Design review of the part built by this model. Coordinates are the model's own, in mm. A direction names the side the tool comes from. Coordinates: 2 decimals unless noted, no trailing zeros. Loops run counter-clockwise (first coordinate to the right, second up) from the corner with the lowest first, then second, coordinate; pieces in that order, holes last. Notation, with made-up numbers: (13, 22.25) - (55, 22.25) arc R34 cw to (55, 55.25) - close; hole circle Ø8 at (43.5, -13.75). An arc over 180 degrees is marked (long way). Answer in a Markdown table with one row per item. Add a question column.
(1) To check wall thickness, follow L1, parallel to Y at x = 82, z = 45.5; L2, parallel to Y at x = -76, z = 28; L3, parallel to Z at x = 85, y = -9.5. State the ranges of each line that lie inside material, in increasing order. Write a range as [from, to].
(2) The part is to be moulded in two halves that separate along X. For faces 3 (the face through (-53.978, -5.67, -133.786)), 4 (the face through (-79.557, 3.451, -113.968)), 5 (the face through (-113, 0, 112)), 6 (the face through (55.637, -5.67, 110.036)), say which applies: released by +X, released by -X, zero draft, split by the parting line, or undercut.
(3) We need section A-A, the plane y = 3.5. Write out the cut boundary in (x, z), plus the area to 3 significant figures.
(4) For faces 1 (the face through (-78, 0, -2)), 2 (the face through (-55, 8, 34)), list the 3-axis set-ups (+Z, -Z, +X, -X, +Y, -Y) from which the entire face can be reached by the end or side of a thin tool; tool diameter is ignored.
(5) Clearance check with flat-ended pins moving along their axes: pin 1 (1 mm diameter, centred on y = -8, z = 42, fed in from -X); pin 2 (8 mm diameter, centred on y = 4.5, z = 80, fed in from -X); pin 3 (4 mm diameter, centred on y = -7.5, z = 12.5, fed in from -X); pin 4 (11.5 mm diameter, centred on x = -53.13, z = -140.23, fed in from +Y). State where each tip first meets the part, or that it passes through.
from build123d import *

# Parameters (mm, degrees)
F0_R     = 160
F0_R_2   = 6.5
F0_R_3   = 36
F1_DEPTH = 11.5
F2_SIZE  = 1
F3_R     = 122
F3_R_2   = 36
F3_R_3   = 25.5
F4_DEPTH = 8
F5_SIZE  = 1


with BuildPart() as f1:
    # F0 (on Front) → F1 (new body)
    with BuildSketch(Plane.XZ):
        with Locations((-53.132202721, 5.1132893958)):
            Circle(F0_R)
        with Locations((-155.6978265414, -97.8607830485)):
            Circle(F0_R_2, mode=Mode.SUBTRACT)
        with Locations((-53.132202721, -140.2307106042)):
            Circle(F0_R_2, mode=Mode.SUBTRACT)
        with Locations((49.4334210995, -97.8607830485)):
            Circle(F0_R_2, mode=Mode.SUBTRACT)
        with Locations((90.8079806329, 5.1103962891)):
            Circle(F0_R_2, mode=Mode.SUBTRACT)
        with Locations((-197.0651851107, 5.1132893958)):
            Circle(F0_R_2, mode=Mode.SUBTRACT)
        with Locations((-155.6978265414, 108.08736184)):
            Circle(F0_R_2, mode=Mode.SUBTRACT)
        with Locations((-53.132202721, 5.1132893958)):
            Circle(F0_R_3, mode=Mode.SUBTRACT)
        with Locations((-53.132202721, 150.4572893958)):
            Circle(F0_R_2, mode=Mode.SUBTRACT)
        with Locations((49.4375604441, 108.0832387485)):
            Circle(F0_R_2, mode=Mode.SUBTRACT)
    extrude(amount=F1_DEPTH)

    # F2
    f2_edges = [f1.edges().sort_by_distance(p)[0] for p in [
        (-213.132203, 0, 5.113289),
        (-213.132203, -11.5, 5.113289),
    ]]
    chamfer(f2_edges, length=F2_SIZE)

    # F3 (on face) → F4 (join)
    with BuildSketch(Plane.XZ):
        with Locations((-53.1101636589, 5.1305745728)):
            Circle(F3_R)
        with Locations((-53.132202721, 5.1132893958)):
            Circle(F3_R_2, mode=Mode.SUBTRACT)
        with Locations((-53.132202721, 5.1132893958)):
            Circle(F3_R_2)
        with Locations((-53.1101636589, 5.1305745728)):
            Circle(F3_R_3, mode=Mode.SUBTRACT)
    extrude(amount=-F4_DEPTH)

    # F5
    f5_edges = [f1.edges().sort_by_distance(p)[0] for p in [
        (-175.110164, 8, 5.130575),
    ]]
    chamfer(f5_edges, length=F5_SIZE)


solid = f1.part
Responses:
| question | item | result |
|---|---|---|
| 1 | L1 | y = [-11.5, 0] |
| 1 | L2 | y = [0, 8] |
| 1 | L3 | z = [-75.63, 2.19], [8.03, 85.86] |
| 2 | face 3 | undercut |
| 2 | face 4 | split by the parting line |
| 2 | face 5 | zero draft |
| 2 | face 6 | undercut |
| 3 | outline | circle Ø244 at (-53.11, 5.13); hole circle Ø51 at (-53.11, 5.13) |
| 3 | area | 44,700 mm2 |
| 4 | face 1 | -Y |
| 4 | face 2 | +Z, -Z, +X, -X, +Y |
| 5 | pin 1 | stops at x = -208.94 |
| 5 | pin 2 | stops at x = -152.42 |
| 5 | pin 3 | stops at x = -213.04 |
| 5 | pin 4 | passes through |
